Study the drawing (mm; zero at the part's minimum x, y, z) and answer. Coordinates: 2 decimals unless noted, no trailing zeros. Order: outer loops, then holes, each group sorted by start corner. A loop starts at its lowest first (then second) coordinate and runs counter-clockwise, first axis right, second up. Notation, with made-up numbers: (7, 66.25) -> (11, 66.25) arc R14 ccw to (11, 70.25) -> close; hole circle Ø8 at (89, 9). An arc over 180 degrees is marked (long way). Answer in a Markdown table with one row per item. Add a question column.
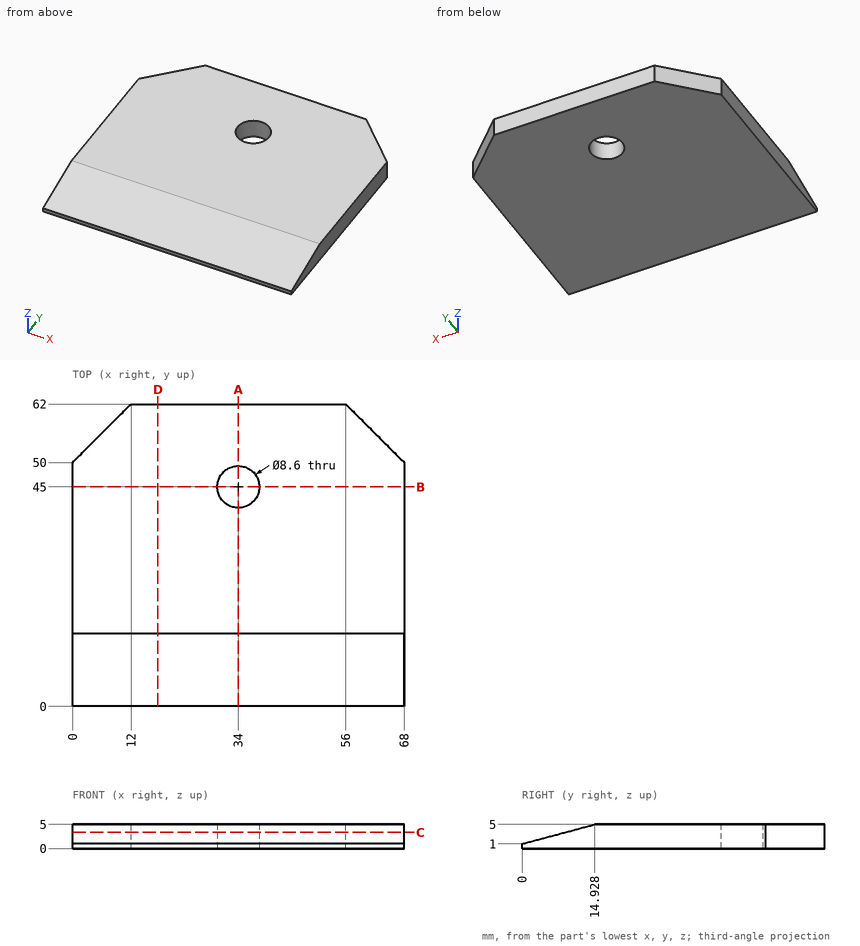
Q1. A cutting plane is placed at B-B (y = 45). Determine the outline of the cut face in (x, z), then the cut area to 3 significant figures.
Q2. Straight lines are drawn through the part: line 1 (X direction, y = 59.5, z = 0.8); line 2 (Z direction, x = 54, y = 9); line 3 (X direction, y = 46.5, z = 4.1). For each, find the intervals that lie inside material, in ascending order.
Q3. A cutting plane is placed at D-D (x = 17.5). Determine the outline of the cut face in (y, z).
Q4. A cutting plane is placed at C-C (z = 3.35). Determine the outline of the cut face in (x, y), then the cut area to 3 significant figures.
Q5. A cutting plane is placed at A-A (x = 34). Determine the outline of the cut face in (y, z), then the cut area to 3 significant figures.
Returned:
| question | item | result |
|---|---|---|
| 1 | outline | (0, 0) -> (29.7, 0) -> (29.7, 5) -> (0, 5) -> close; (38.3, 0) -> (68, 0) -> (68, 5) -> (38.3, 5) -> close |
| 1 | area | 297 mm² |
| 2 | line 1 | x = 9.5 to 58.5 |
| 2 | line 2 | z = 0 to 3.41 |
| 2 | line 3 | x = 0 to 29.97, 38.03 to 68 |
| 3 | outline | (0, 0) -> (62, 0) -> (62, 5) -> (14.93, 5) -> (0, 1) -> close |
| 4 | outline | (0, 8.77) -> (68, 8.77) -> (68, 50) -> (56, 62) -> (12, 62) -> (0, 50) -> close; hole circle Ø8.6 at (34, 45) |
| 4 | area | 3,420 mm² |
| 5 | outline | (0, 0) -> (40.7, 0) -> (40.7, 5) -> (14.93, 5) -> (0, 1) -> close; (49.3, 0) -> (62, 0) -> (62, 5) -> (49.3, 5) -> close |
| 5 | area | 237 mm² |
